Check sheet for the modelled part. Datum: model origin and axes. Units: mm. A direction names the side the tool comes from. Round coordinates to 2 decimals unless told otherwise and drop trailing zeros. Write each loop counter-clockwise with the first axis right and the second up, starting at its lowest first coordinate (ties: lowest second). Pieces come first, ordered by that corner, then holes.
Item 1: Cross-section at B-B on z = 3.75. Enter the section's corners in (x, y).
Item 2: Cross-section at D-D on x = 3.75. Enter the section's corners in (y, z), plus the area to 3 significant figures.
Item 3: Go/stop test with flat-tipped pins: pin 1 Ø8 at (y, z) = (6.5, 13) entering from +X; pin 2 Ø3 at (x, y) = (-10.57, 22.66) entering from +Z; pin 3 Ø10 at (y, z) = (18, 6) entering from +X; pin 4 Ø12 at (y, z) = (12.5, 5.5) entering from +X. Record where each tip stops, or that it passes through.
Item 4: Release check for a two-part mould opening along X. For faces 4 (the cylindrical face through (-10, 21, 4)), 5 (the flat face through (-0.825, 13.601, 3.698)), 6 (the cylindrical face through (-12.18, 27.39, 19.53)) record: +X half, -X half, draft (parallel to the pull), parting line (faces both ways), or undercut.
Item 5: Material ranges on line 1 (Z direction, x = -5.25, y = 19.5); line 2 (Y direction, x = 6.75, z = 8.25); line 3 (X direction, y = 1.5, z = 18), recorded low to high.
Item 6: Cross-section at C-C on y = -25. Enter the section's corners in (x, z).
Item 7: Tool access check on faces 1 (the flat face through (7.5, -26, 12)), 2 (the flat face through (6, -17.5, 12)), 3 (the flat face through (-3, -5, 12)). Record the directions out of +Z, -Z, +X, -X, +Y, -Y that give a thin tool (end or side, any length) a straight path to the whole face; none if there is none.
Item 8: Cross-section at A-A on x = 0. Enter the section's corners in (y, z), plus the area to 3 significant figures.
from build123d import *

# Parameters (mm, degrees)
SKETCH1_R           = 1.75
BOSS_EXTRUDE1_DEPTH = 7.5
BOSS_EXTRUDE2_DEPTH = 8.333333333
SKETCH3_R           = 1.75
BOSS_EXTRUDE4_DEPTH = 7.5
SKETCH4_W           = 23.333333333
SKETCH4_H           = 17.5
BOSS_EXTRUDE5_DEPTH = 2.5


with BuildPart() as part:
    # Sketch1 → Boss-Extrude1 (new body)
    with BuildSketch(Plane.XY):
        with BuildLine():
            Line((-6.033917608, 24.770785985), (4.531538935, 2.113091309))
            ThreePointArc((4.531538935, 2.113091309), (4.881480036, 1.08219807), (5, 0))
            Line((5, 0), (5, -35))
            Line((5, -35), (-5.1028501, -35))
            Line((-5.1028501, -35), (-15.483867589, 21.758121008))
            ThreePointArc((-15.483867589, 21.758121008), (-12.084158316, 27.421468907), (-6.033917608, 24.770785985))
        make_face()
        with Locations((-10.565456544, 22.657694676)):
            Circle(SKETCH1_R, mode=Mode.SUBTRACT)
        Circle(SKETCH1_R, mode=Mode.SUBTRACT)
    extrude(amount=BOSS_EXTRUDE1_DEPTH)

    # Sketch2 → Boss-Extrude2 (add)
    with BuildSketch(Plane.XY.offset(7.5)):
        Polygon((5, -5), (-10.589827455, -5), (-5.1028501, -35), (5, -35), align=None)
    extrude(amount=BOSS_EXTRUDE2_DEPTH)

    # Sketch3 → Boss-Extrude4 (add)
    with BuildSketch(Plane.XY.offset(15.833333333)):
        with BuildLine():
            Line((5, 0), (5, -35))
            Line((5, -35), (-5.1028501, -35))
            Line((-5.1028501, -35), (-15.483867589, 21.758121008))
            ThreePointArc((-15.483867589, 21.758121008), (-12.084158316, 27.421468907), (-6.033917608, 24.770785985))
            Line((-6.033917608, 24.770785985), (4.531538935, 2.113091309))
            ThreePointArc((4.531538935, 2.113091309), (4.881480036, 1.08219807), (5, 0))
        make_face()
        Circle(SKETCH3_R, mode=Mode.SUBTRACT)
        with Locations((-10.565456544, 22.657694676)):
            Circle(SKETCH3_R, mode=Mode.SUBTRACT)
    extrude(amount=BOSS_EXTRUDE4_DEPTH)

    # Sketch4 → Boss-Extrude5 (add)
    with BuildSketch(Plane(origin=(5, 0, 0), x_dir=(0, 0, -1), z_dir=(1, 0, 0))):
        with Locations((-11.666666667, -26.25)):
            Rectangle(SKETCH4_W, SKETCH4_H)
    extrude(amount=BOSS_EXTRUDE5_DEPTH)


solid = part.part
Response values:
1. outline: (-15.48, 21.76) - (-5.1, -35) - (7.5, -35) - (7.5, -17.5) - (5, -17.5) - (5, 0) arc R5 ccw to (4.53, 2.11) - (-6.03, 24.77) arc R5 ccw to start; hole circle Ø3.5 at (-10.57, 22.66); hole circle Ø3.5 at (0, 0)
2. outline: (-35, 0) - (3.79, 0) - (3.79, 7.5) - (-5, 7.5) - (-5, 15.83) - (3.79, 15.83) - (3.79, 23.33) - (-35, 23.33) - close
2. area: 832 mm2
3. pin 1: stops at x = 3.8
3. pin 2: passes through
3. pin 3: stops at x = -0.55
3. pin 4: stops at x = 2.49
4. face 4: undercut
4. face 5: +X half
4. face 6: parting line
5. line 1: z = 0 to 7.5, 15.83 to 23.33
5. line 2: y = -35 to -17.5
5. line 3: x = -11.78 to -0.9, 0.9 to 4.77
6. outline: (-6.93, 0) - (7.5, 0) - (7.5, 23.33) - (-6.93, 23.33) - close
7. face 1: +Z, -Z, +X, +Y, -Y
7. face 2: +Z, -Z, +X, +Y
7. face 3: +X, -X, +Y
8. outline: (-35, 0) - (-1.75, 0) - (-1.75, 7.5) - (-5, 7.5) - (-5, 15.83) - (-1.75, 15.83) - (-1.75, 23.33) - (-35, 23.33) - close; (1.75, 0) - (11.83, 0) - (11.83, 7.5) - (1.75, 7.5) - close; (1.75, 15.83) - (11.83, 15.83) - (11.83, 23.33) - (1.75, 23.33) - close
8. area: 900 mm2
